Geometry check sheet. Reference: drawing and pictorial views, mm from the part's lowest x, y, z. Round coordinates to 2 decimals unless told otherwise and drop trailing zeros. Order: outer loops, then holes, each group sorted by start corner. A loop starts at its lowest first (then second) coordinate and runs counter-clockwise, first axis right, second up.
(1) Depth check by flat-ended pin: pin 1 (3.5 mm diameter, centred on x = 17.5, y = 17.5, fed in from +Z); pin 2 (1.5 mm diameter, centred on x = 12.5, z = 5, fed in from -Y); pin 3 (2 mm diameter, centred on x = 14, z = 9, fed in from -Y). Enter the tip coordinate at first touch or a pass-through.
(2) Mould release check, pull along X, two halves, no side actions. Record for the marked faces 1, 2 and 3: released by +X, released by -X, zero draft, split by the parting line, or undercut.
(3) Sectioned sample at A-A, the plane z = 8.5. Enter the section's corners in (x, y).
(4) Thickness scan on probe 1 along Y at (x, z) = (17.5, 6.5); probe 2 along Y at (x, z) = (17.5, 2.3); probe 3 along X at (y, z) = (15, 15.5). Record the ranges inside material, lowest first.
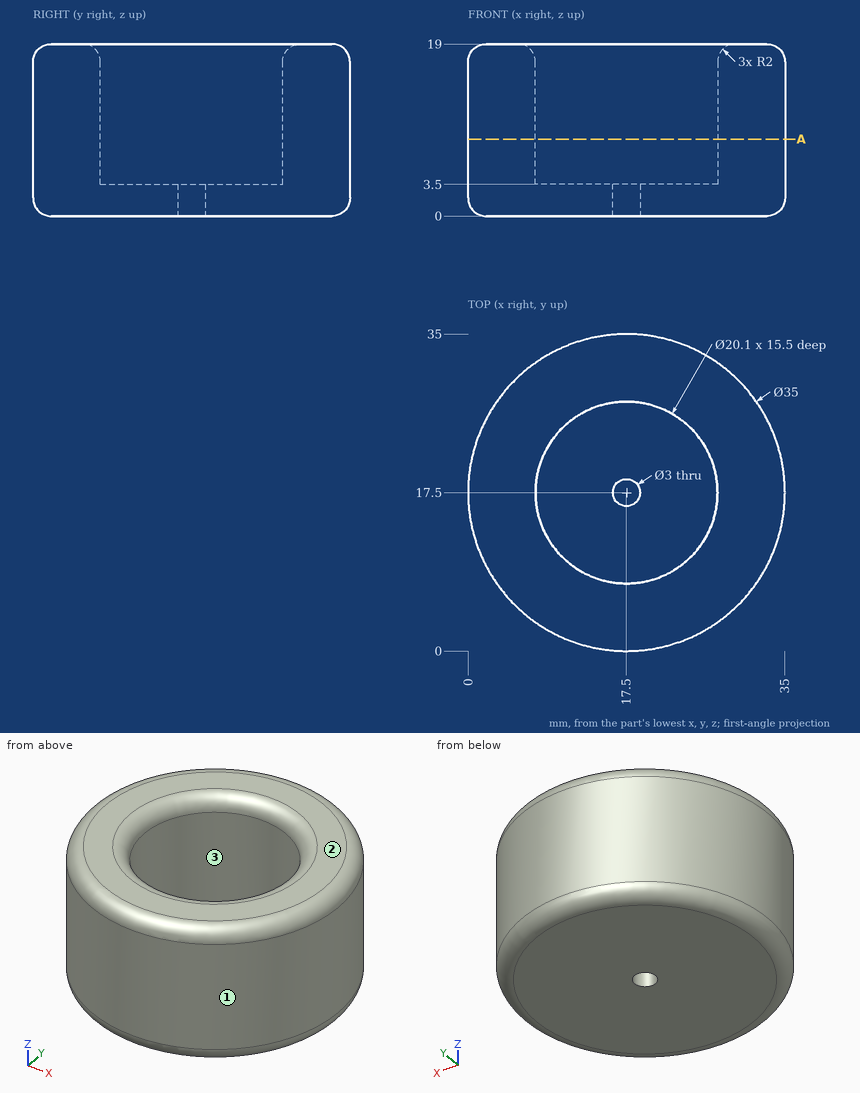
Derived:
1. pin 1: stops at z = 3.5
1. pin 2: stops at y = 0.52
1. pin 3: stops at y = 0.18
2. face 1: split by the parting line
2. face 2: zero draft
2. face 3: undercut
3. outline: circle Ø35 at (17.5, 17.5); hole circle Ø20.1 at (17.5, 17.5)
4. probe 1: y = 0 to 7.45, 27.55 to 35
4. probe 2: y = 0 to 16, 19 to 35
4. probe 3: x = 0.18 to 7.77, 27.23 to 34.82
